Here's how the part is built. I have some questions about the finished solid (model axes, mm). Round coordinates to 2 decimals unless told otherwise and drop trailing zeros. Loops run counter-clockwise (first coordinate to the right, second up) from the corner with the lowest first, then second, coordinate; pieces in that order, holes last. Notation, with made-up numbers: M 29.25,37.5 L 71.25,37.5 A8 cw 71.25,45.5 Z; hole C 26,22 d10. An arc over 180 degrees is marked long. Write each question's results on one line, items separated by ' | '. Start each with the question number.
```python
from build123d import *

# Parameters (mm, degrees)
ESTRUSIONE_ESTRUSIONE1_DEPTH = 20
SCHIZZO5_R                   = 3
TAGLIO_ESTRUSIONE1_DEPTH     = 144.181702742


with BuildPart() as part:
    # Schizzo1 → Estrusione-Estrusione1 (new body)
    with BuildSketch(Plane.XY):
        Polygon((60, 126), (60, -126), (-65, -126), (-65, 126), (-60, 126), align=None)
    extrude(amount=ESTRUSIONE_ESTRUSIONE1_DEPTH)

    # Schizzo5 → Taglio-Estrusione1 (cut, through all)
    with BuildSketch(Plane(origin=(0, 0, 0), x_dir=(-1, 0, 0), z_dir=(0, 0, -1))):
        with Locations((51, 108)):
            Circle(SCHIZZO5_R)
        with Locations((51, 63)):
            Circle(SCHIZZO5_R)
        with Locations((-6, 108)):
            Circle(SCHIZZO5_R)
        with Locations((-6, 63)):
            Circle(SCHIZZO5_R)
        with Locations((11.000000001, 22.499999999)):
            Circle(SCHIZZO5_R)
        with Locations((11.000000001, -22.500000001)):
            Circle(SCHIZZO5_R)
        with Locations((-45.999999999, 22.499999999)):
            Circle(SCHIZZO5_R)
        with Locations((-45.999999999, -22.500000001)):
            Circle(SCHIZZO5_R)
        with Locations((-6, -63)):
            Circle(SCHIZZO5_R)
        with Locations((-6, -108)):
            Circle(SCHIZZO5_R)
        with Locations((51, -63)):
            Circle(SCHIZZO5_R)
        with Locations((51, -108)):
            Circle(SCHIZZO5_R)
    extrude(amount=-TAGLIO_ESTRUSIONE1_DEPTH, mode=Mode.SUBTRACT)


solid = part.part
```
Item 1: If we section it at B-B on y = -22.5: Please give me the cut outline in (x, z), and give its area (3 significant figures).
Item 2: I'm going to push a flat-ended pin straight in: pin 1 (5.5 mm diameter, centred on x = -51, y = -63, fed in from -Z). Where does the tip first touch, or does it pass through?
Item 3: If we mould it in two halves opening along Y, with no side actions, what happens to faces 1 (the face through (-2, -126, 10)), 2 (the face through (-65, -2, 10)), 3 (the face through (6.65, 105.07, 9.86)), 4 (the face through (-2, 126, 10))? For each: released by +Y, released by -Y, zero draft, split by the parting line, or undercut.
Item 4: I need wall thicknesses on L1, parallel to Y at x = 6, z = 13.5; L2, parallel to Y at x = 46, z = 10.5; L3, parallel to X at y = 61, z = 2. Which ranges of each line are inside material? Lowest first, please.
Item 5: If we section it at A-A on x = 46: Please give me the cut outline in (y, z).
Item 6: If we section it at C-C on x = -50.5: Please give me the cut outline in (y, z), and give its area (3 significant figures).
Numbers:
1) outline: M -65,0 L -14,0 L -14,20 L -65,20 Z; M -8,0 L 43,0 L 43,20 L -8,20 Z; M 49,0 L 60,0 L 60,20 L 49,20 Z | area: 2,260 mm²
2) pin 1: through
3) face 1: released by -Y | face 2: zero draft | face 3: undercut | face 4: released by +Y
4) L1: -126 to -111, -105 to -66, -60 to 60, 66 to 105, 111 to 126 | L2: -126 to -25.5, -19.5 to 19.5, 25.5 to 126 | L3: -65 to -53.24, -48.76 to 3.76, 8.24 to 60
5) outline: M -126,0 L -25.5,0 L -25.5,20 L -126,20 Z; M -19.5,0 L 19.5,0 L 19.5,20 L -19.5,20 Z; M 25.5,0 L 126,0 L 126,20 L 25.5,20 Z
6) outline: M -126,0 L -110.96,0 L -110.96,20 L -126,20 Z; M -105.04,0 L -65.96,0 L -65.96,20 L -105.04,20 Z; M -60.04,0 L 60.04,0 L 60.04,20 L -60.04,20 Z; M 65.96,0 L 105.04,0 L 105.04,20 L 65.96,20 Z; M 110.96,0 L 126,0 L 126,20 L 110.96,20 Z | area: 4,570 mm²
